```python
from build123d import *

# Parameters (mm, degrees)
SKETCH2_R               = 5
BOSS_EXTRUDE1_DEPTH     = 10
BOSS_EXTRUDE2_DEPTH     = 5
CUT_EXTRUDE1_DEPTH      = 64.079315152
CUT_EXTRUDE1_DEPTH_BACK = 64.079315152
SKETCH4_R               = 2.5
SKETCH5_R               = 6
CUT_EXTRUDE2_DEPTH      = 2.5
CUT_EXTRUDE3_DEPTH      = 2.5
CUT_EXTRUDE3_DEPTH_BACK = 2.5
SKETCH7_R               = 8.5
SKETCH9_RX              = 3.80806065
SKETCH9_RY              = 2.813161922
CUT_EXTRUDE4_DEPTH      = 2
CUT_EXTRUDE5_DEPTH      = 2
SKETCH12_R              = 0.65
CUT_EXTRUDE6_DEPTH      = 63.633856702
CUT_EXTRUDE7_DEPTH      = 63.633856702


with BuildPart() as part:
    # Sketch2 → Boss-Extrude1 (new, symmetric)
    with BuildSketch(Plane.XY):
        Circle(SKETCH2_R)
    extrude(amount=BOSS_EXTRUDE1_DEPTH, both=True)

    # Sketch3 → Boss-Extrude2 (add, symmetric)
    with BuildSketch(Plane.XY):
        with BuildLine():
            Line((1, 4.898979486), (5, 34))
            Line((5, 34), (0, 34))
            Line((0, 34), (0, 40))
            ThreePointArc((0, 40), (7.071067812, 42.928932188), (10, 50))
            ThreePointArc((10, 50), (14.673051661, 54.989299027), (19.957241913, 50.652497212))
            Line((19.957241913, 50.652497212), (26.957241913, -2.528869287))
            ThreePointArc((26.957241913, -2.528869287), (22.326948339, -8.170665526), (17, -3.181366499))
            Line((17, -3.181366499), (3.857318654, -3.181366499))
            Line((3.857318654, -3.181366499), (1, 4.898979486))
        make_face()
    extrude(amount=BOSS_EXTRUDE2_DEPTH, both=True)

    # Sketch4 → Cut-Extrude1 (cut, two sides: drawn at the far end of the back side and taken through both)
    with BuildSketch(Plane.XY.offset(5).offset(-CUT_EXTRUDE1_DEPTH_BACK)):
        with Locations((15, 50)):
            Circle(SKETCH4_R)
        Circle(SKETCH4_R)
        with Locations((22, -3.181366499)):
            Circle(SKETCH4_R)
    extrude(amount=CUT_EXTRUDE1_DEPTH + CUT_EXTRUDE1_DEPTH_BACK, mode=Mode.SUBTRACT)

    # Sketch5 → Cut-Extrude2 (cut)
    with BuildSketch(Plane.XY.offset(5)):
        with Locations((15, 50)):
            Circle(SKETCH5_R)
    cut_extrude2 = extrude(amount=-CUT_EXTRUDE2_DEPTH, mode=Mode.SUBTRACT)

    # Mirror1: Cut-Extrude2 across plane
    add(cut_extrude2.mirror(Plane.XY), mode=Mode.SUBTRACT)

    # Sketch7 → Cut-Extrude3 (cut, two sides: drawn at the far end of the back side and taken through both)
    with BuildSketch(Plane.XY.offset(-CUT_EXTRUDE3_DEPTH_BACK)):
        with Locations((22, -3.181366499)):
            Circle(SKETCH7_R)
    extrude(amount=CUT_EXTRUDE3_DEPTH + CUT_EXTRUDE3_DEPTH_BACK, mode=Mode.SUBTRACT)

    # Sketch9 → Cut-Extrude4 (cut)
    with BuildSketch(Plane.XY.offset(5)):
        with Locations(Location((13.227873683, 18.281882493), (0, 0, 90))):
            Ellipse(SKETCH9_RX, SKETCH9_RY)
    cut_extrude4 = extrude(amount=-CUT_EXTRUDE4_DEPTH, mode=Mode.SUBTRACT)

    # Sketch11 → Cut-Extrude5 (cut)
    with BuildSketch(Plane.XY.offset(5)):
        with BuildLine():
            add(Edge.make_bspline(
                [(12.522028797, 21.968126834), (12.172187814, 21.786407618), (10.359411342, 23.317925648), (11.369156283, 27.907682858), (13.176267664, 22.307960587), (12.522028797, 21.968126834)],
                knots=[0, 0, 0, 0, 0.25167876, 0.529334656, 1, 1, 1, 1], degree=3))
        make_face()
        with BuildLine():
            add(Edge.make_bspline(
                [(13.933718568, 21.968126834), (14.276902775, 21.772094059), (16.056700712, 23.2943812), (15.069290945, 27.627740223), (13.320756239, 22.318261556), (13.933718568, 21.968126834)],
                knots=[0, 0, 0, 0, 0.263421901, 0.529501361, 1, 1, 1, 1], degree=3))
        make_face()
    cut_extrude5 = extrude(amount=-CUT_EXTRUDE5_DEPTH, mode=Mode.SUBTRACT)

    # Sketch12 → Cut-Extrude6 (cut, through all)
    with BuildSketch(Plane.XY.offset(3)):
        with Locations((12.466071171, 19.745676536)):
            Circle(SKETCH12_R)
        with Locations((13.933718568, 19.745676536)):
            Circle(SKETCH12_R)
    extrude(amount=-CUT_EXTRUDE6_DEPTH, mode=Mode.SUBTRACT)

    # Sketch13 → Cut-Extrude7 (cut, through all)
    with BuildSketch(Plane.XY.offset(3)):
        with BuildLine():
            Line((11.848135132, 17.156912107), (14.607612233, 17.156912107))
            ThreePointArc((14.607612233, 17.156912107), (13.227873683, 15.777173557), (11.848135132, 17.156912107))
        make_face()
    extrude(amount=-CUT_EXTRUDE7_DEPTH, mode=Mode.SUBTRACT)

    # Mirror2: Cut-Extrude4, Cut-Extrude5 across plane
    add(cut_extrude4.mirror(Plane.XY), mode=Mode.SUBTRACT)
    add(cut_extrude5.mirror(Plane.XY), mode=Mode.SUBTRACT)


solid = part.part
```
For this review, take the finished solid that the model builds, in its own axes (mm). A direction names the side the tool comes from. Coordinates: 2 decimals unless noted, no trailing zeros. Write each loop counter-clockwise with the first axis right and the second up, starting at its lowest first coordinate (ties: lowest second). Pieces come first, ordered by that corner, then holes. Notation, with made-up numbers: (-1, -21.75) - (24, -21.75) arc R20 cw to (24, -8.75) - close; hole circle Ø6 at (-27.75, 23.5). An arc over 180 degrees is marked (long way). Answer in a Markdown table with one row per item. Add a question column.
Q1. We need section B-B, the plane z = -0.75. State the section outline as (x, y) points.
Q2. Draft analysis for pull direction Y (two halves, no side actions). For faces 1 (the flat face through (2, -2, 10)), 2 (the flat face through (2.972, 19.246, 0.07)), 3 (the cylindrical face through (15, 44, 4)), state which applies: +Y half, -Y half, draft (parallel to the pull), parting line (faces both ways), or undercut.
Q3. For probe 1 along Y at (x, z) = (14.5, 4.75); probe 2 along Z at (x, y) = (25, -6), list the stretches that pass through material, from the lowest coordinate up.
Q4. Tool access review of faces 4 (the cylindrical face through (17.762, 4.187, -0.035)), 5 (the flat face through (13, 17.157, 0)), 6 (the cylindrical face through (6.99, 42.85, 0.07)), 7 (the flat face through (3, 34, 0)), 8 (the flat face through (2, -2, -10)): name each direction out of +Z, -Z, +X, -X, +Y, -Y from which nothing blocks a thin tool from reaching the whole face with its end or side.
Q5. For P1, Ø3, axis at x = 14, y = 49.5, coming from the +Z side; P2, Ø8, axis at x = -1.5, y = 30, coming from the -Z side; P3, Ø3, axis at y = 38.5, z = 0.5, coming from the -X side; P4, Ø1, axis at x = 20, y = 38.5, coming from the +Z side, all flat-tipped, find the tip position at first contact; note any pin that passes through.
Q6. We need section A-A, the plane y = -4. State the section outline as (x, z) points.
Q7. We need section C-C, the plane x = 21. State the section outline as (y, z) points, and give its area (3 significant figures).
Q8. We need section D-D, the plane z = 8.25. State the section outline as (x, y) points, and give its area (3 significant figures).
Answer list:
| question | item | result |
|---|---|---|
| 1 | outline | (0, 34) - (5, 34) - (1, 4.9) arc R5 ccw (long way) to (3.86, -3.18) - (13.5, -3.18) arc R8.5 cw to (26.06, 4.29) - (19.96, 50.65) arc R5 ccw to (10, 50) arc R10 cw to (0, 40) - close; hole circle Ø5 at (0, 0); hole circle Ø1.3 at (12.47, 19.75); hole (11.85, 17.16) arc R1.38 ccw to (14.61, 17.16) - close; hole circle Ø5 at (15, 50); hole circle Ø1.3 at (13.93, 19.75) |
| 2 | face 1 | draft |
| 2 | face 2 | undercut |
| 2 | face 3 | +Y half |
| 3 | probe 1 | y = -3.18 to 14.89, 21.68 to 22.12, 25.03 to 44.02 |
| 3 | probe 2 | z = -5 to -2.5, 2.5 to 5 |
| 4 | face 4 | -Y |
| 4 | face 5 | +Z, -Z |
| 4 | face 6 | +Z, -Z, -X, +Y |
| 4 | face 7 | +Z, -Z, -X |
| 4 | face 8 | -Z, +X, -X, +Y, -Y |
| 5 | P1 | stops at z = 2.5 |
| 5 | P2 | passes through |
| 5 | P3 | stops at x = 0 |
| 5 | P4 | stops at z = 5 |
| 6 | outline | (-3, -10) - (3, -10) - (3, 10) - (-3, 10) - close; (17.07, -5) - (19.64, -5) - (19.64, -2.5) - (17.07, -2.5) - close; (17.07, 2.5) - (19.64, 2.5) - (19.64, 5) - (17.07, 5) - close; (24.36, -5) - (26.93, -5) - (26.93, -2.5) - (24.36, -2.5) - close; (24.36, 2.5) - (26.93, 2.5) - (26.93, 5) - (24.36, 5) - close |
| 7 | outline | (-8.08, -5) - (-5.47, -5) - (-5.47, -2.5) - (-8.08, -2.5) - close; (-8.08, 2.5) - (-5.47, 2.5) - (-5.47, 5) - (-8.08, 5) - close; (-0.89, -5) - (42.73, -5) - (42.73, 5) - (-0.89, 5) - (-0.89, 2.5) - (5.26, 2.5) - (5.26, -2.5) - (-0.89, -2.5) - close |
| 7 | area | 418 mm2 |
| 8 | outline | circle Ø10 at (0, 0); hole circle Ø5 at (0, 0) |
| 8 | area | 58.9 mm2 |
